from build123d import *

# Parameters (mm, degrees)
F1_DEPTH = 6.35


with BuildPart() as f1:
    # F0 (on Top) → F1 (new body)
    with BuildSketch(Plane.XY):
        with BuildLine():
            ThreePointArc((57.94375, -25.976370723), (48.024670033, -14.636026826), (44.45, 0))
            ThreePointArc((44.45, 0), (0, -44.45), (-44.45, 0))
            ThreePointArc((-44.45, 0), (-48.024670033, -14.636026826), (-57.94375, -25.976370723))
            ThreePointArc((-57.94375, -25.976370723), (-53.0122296555, -34.9564515783), (-46.7007710297, -43.0265962543))
            ThreePointArc((-46.7007710297, -43.0265962543), (-46.1408199964, -43.6066686624), (-45.5932687094, -44.1984597966))
            ThreePointArc((-45.5932687094, -44.1984597966), (0, -63.5), (45.5932687094, -44.1984597966))
            ThreePointArc((45.5932687094, -44.1984597966), (46.1408199964, -43.6066686624), (46.7007710297, -43.0265962543))
            ThreePointArc((46.7007710297, -43.0265962543), (53.0122296555, -34.9564515783), (57.94375, -25.976370723))
        make_face()
        with BuildLine():
            ThreePointArc((57.94375, 25.976370723), (48.024670033, 14.636026826), (44.45, 0))
            Line((44.45, 0), (63.5, 0))
            ThreePointArc((63.5, 0), (62.0954029096, 13.2819779212), (57.94375, 25.976370723))
        make_face()
        with BuildLine():
            ThreePointArc((-44.45, 0), (0, 44.45), (44.45, 0))
            ThreePointArc((44.45, 0), (48.024670033, 14.636026826), (57.94375, 25.976370723))
            ThreePointArc((57.94375, 25.976370723), (53.0122296555, 34.9564515783), (46.7007710297, 43.0265962543))
            ThreePointArc((46.7007710297, 43.0265962543), (46.1408199964, 43.6066686624), (45.5932687094, 44.1984597966))
            ThreePointArc((45.5932687094, 44.1984597966), (0, 63.5), (-45.5932687094, 44.1984597966))
            ThreePointArc((-45.5932687094, 44.1984597966), (-46.1408199964, 43.6066686624), (-46.7007710297, 43.0265962543))
            ThreePointArc((-46.7007710297, 43.0265962543), (-53.0122296555, 34.9564515783), (-57.94375, 25.976370723))
            ThreePointArc((-57.94375, 25.976370723), (-48.024670033, 14.636026826), (-44.45, 0))
        make_face()
        with BuildLine():
            Line((63.5, 0), (44.45, 0))
            ThreePointArc((44.45, 0), (48.024670033, -14.636026826), (57.94375, -25.976370723))
            ThreePointArc((57.94375, -25.976370723), (62.0954029096, -13.2819779212), (63.5, 0))
        make_face()
        with BuildLine():
            ThreePointArc((-57.94375, -25.976370723), (-48.024670033, -14.636026826), (-44.45, 0))
            Line((-44.45, 0), (-63.5, 0))
            ThreePointArc((-63.5, 0), (-62.0954029096, -13.2819779212), (-57.94375, -25.976370723))
        make_face()
        with BuildLine():
            Line((-63.5, 0), (-44.45, 0))
            ThreePointArc((-44.45, 0), (-48.024670033, 14.636026826), (-57.94375, 25.976370723))
            ThreePointArc((-57.94375, 25.976370723), (-62.0954029096, 13.2819779212), (-63.5, 0))
        make_face()
        with BuildLine():
            ThreePointArc((76.2, -12.7), (67.2197438789, -8.9802561211), (63.5, 0))
            ThreePointArc((63.5, 0), (62.0954029096, -13.2819779212), (57.94375, -25.976370723))
            ThreePointArc((57.94375, -25.976370723), (65.6047024614, -29.9299543947), (74.0468101417, -31.6769044168))
            ThreePointArc((74.0468101417, -31.6769044168), (75.1239218386, -31.6982296864), (76.2, -31.75))
            Line((76.2, -31.75), (76.2, -12.7))
        make_face()
        with BuildLine():
            ThreePointArc((57.94375, 25.976370723), (62.0954029096, 13.2819779212), (63.5, 0))
            ThreePointArc((63.5, 0), (67.2197438789, 8.9802561211), (76.2, 12.7))
            Line((76.2, 12.7), (76.2, 31.75))
            ThreePointArc((76.2, 31.75), (75.1239218386, 31.6982296864), (74.0468101417, 31.6769044168))
            ThreePointArc((74.0468101417, 31.6769044168), (65.6047024614, 29.9299543947), (57.94375, 25.976370723))
        make_face()
        with BuildLine():
            ThreePointArc((46.7007710297, 43.0265962543), (53.0122296555, 34.9564515783), (57.94375, 25.976370723))
            ThreePointArc((57.94375, 25.976370723), (65.6047024614, 29.9299543947), (74.0468101417, 31.6769044168))
            ThreePointArc((74.0468101417, 31.6769044168), (59.2262146143, 34.5867715285), (46.7007710297, 43.0265962543))
        make_face()
        with BuildLine():
            ThreePointArc((74.0468101417, -31.6769044168), (65.6047024614, -29.9299543947), (57.94375, -25.976370723))
            ThreePointArc((57.94375, -25.976370723), (53.0122296555, -34.9564515783), (46.7007710297, -43.0265962543))
            ThreePointArc((46.7007710297, -43.0265962543), (59.2262146143, -34.5867715285), (74.0468101417, -31.6769044168))
        make_face()
        with BuildLine():
            ThreePointArc((-76.2, 12.7), (-67.2197438789, 8.9802561211), (-63.5, 0))
            ThreePointArc((-63.5, 0), (-62.0954029096, 13.2819779212), (-57.94375, 25.976370723))
            ThreePointArc((-57.94375, 25.976370723), (-65.6047024614, 29.9299543947), (-74.0468101417, 31.6769044168))
            ThreePointArc((-74.0468101417, 31.6769044168), (-75.1239218386, 31.6982296864), (-76.2, 31.75))
            Line((-76.2, 31.75), (-76.2, 12.7))
        make_face()
        with BuildLine():
            ThreePointArc((-57.94375, -25.976370723), (-62.0954029096, -13.2819779212), (-63.5, 0))
            ThreePointArc((-63.5, 0), (-67.2197438789, -8.9802561211), (-76.2, -12.7))
            Line((-76.2, -12.7), (-76.2, -31.75))
            ThreePointArc((-76.2, -31.75), (-75.1239218386, -31.6982296864), (-74.0468101417, -31.6769044168))
            ThreePointArc((-74.0468101417, -31.6769044168), (-65.6047024614, -29.9299543947), (-57.94375, -25.976370723))
        make_face()
        with BuildLine():
            ThreePointArc((-74.0468101417, 31.6769044168), (-65.6047024614, 29.9299543947), (-57.94375, 25.976370723))
            ThreePointArc((-57.94375, 25.976370723), (-53.0122296555, 34.9564515783), (-46.7007710297, 43.0265962543))
            ThreePointArc((-46.7007710297, 43.0265962543), (-59.2262146143, 34.5867715285), (-74.0468101417, 31.6769044168))
        make_face()
        with BuildLine():
            ThreePointArc((-46.7007710297, -43.0265962543), (-53.0122296555, -34.9564515783), (-57.94375, -25.976370723))
            ThreePointArc((-57.94375, -25.976370723), (-65.6047024614, -29.9299543947), (-74.0468101417, -31.6769044168))
            ThreePointArc((-74.0468101417, -31.6769044168), (-59.2262146143, -34.5867715285), (-46.7007710297, -43.0265962543))
        make_face()
        with BuildLine():
            Line((76.2, 31.75), (76.2, 12.7))
            ThreePointArc((76.2, 12.7), (85.1802561211, 8.9802561211), (88.9, 0))
            ThreePointArc((88.9, 0), (85.1802561211, -8.9802561211), (76.2, -12.7))
            Line((76.2, -12.7), (76.2, -31.75))
            ThreePointArc((76.2, -31.75), (98.6506403027, -22.4506403027), (107.95, 0))
            ThreePointArc((107.95, 0), (98.6506403027, 22.4506403027), (76.2, 31.75))
        make_face()
        with BuildLine():
            ThreePointArc((-76.2, -12.7), (-88.9, 0), (-76.2, 12.7))
            Line((-76.2, 12.7), (-76.2, 31.75))
            ThreePointArc((-76.2, 31.75), (-107.95, 0), (-76.2, -31.75))
            Line((-76.2, -31.75), (-76.2, -12.7))
        make_face()
    extrude(amount=F1_DEPTH)


solid = f1.part
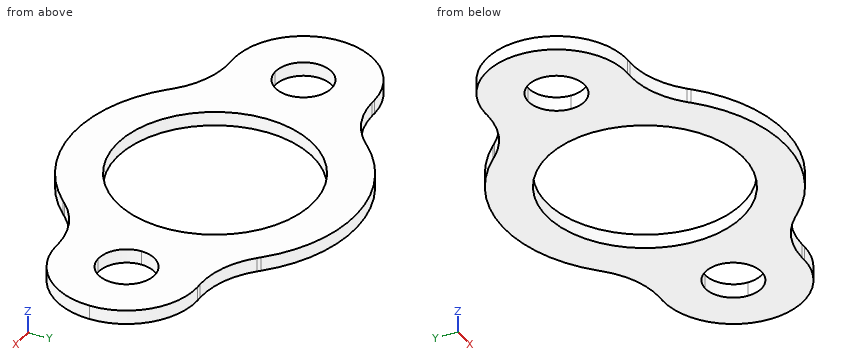
Check sheet for the modelled part. Datum: model origin and axes. Units: mm. Coordinates: 2 decimals unless noted, no trailing zeros. Loops run counter-clockwise (first coordinate to the right, second up) from the corner with the lowest first, then second, coordinate; pieces in that order, holes last. Notation, with made-up numbers: (14.25, 13.25) -> (50.25, 13.25) arc R26 cw to (50.25, 41.25) -> close; hole circle Ø7 at (-27.5, 50.5). An arc over 180 degrees is marked (long way). Write item = value, one per line. Start each with the question number.
1. Depth check by flat-ended pin: P1, Ø1.5, axis at x = 62.5, z = 1, coming from the -Y side; P2, Ø1.5, axis at y = -23.5, z = 5, coming from the +X side; P3, Ø6, axis at x = 31.5, y = 25, coming from the +Z side. Enter the tip coordinate at first touch or a pass-through.
2. Section check A-A on x = 0. Record the cut outline in (y, z), then the cut area to 3 significant figures.
3. Section check B-B on z = 4.5. Record the cut outline in (x, y).
4. Material ranges on line 1 (X direction, y = 9, z = 4.25); line 2 (X direction, y = 9.5, z = 1.5); line 3 (X direction, y = -41, z = 6.25), recorded low to high.
5. Section check D-D on x = 93.5. Record the cut outline in (y, z).
6. Section check C-C on y = 34.5. Record the cut outline in (x, z), then the cut area to 3 significant figures.
Responses:
q1.P1 = -33.64
q1.P2 = 98.35
q1.P3 = through
q2.outline = (-63.5, 0) -> (-44.45, 0) -> (-44.45, 6.35) -> (-63.5, 6.35) -> close; (44.45, 0) -> (63.5, 0) -> (63.5, 6.35) -> (44.45, 6.35) -> close
q2.area = 242 mm2
q3.outline = (-76.2, -31.75) arc R38.1 cw to (-45.59, -44.2) arc R63.5 ccw to (45.59, -44.2) arc R38.1 cw to (76.2, -31.75) arc R31.75 ccw to (76.2, 31.75) arc R38.1 cw to (45.59, 44.2) arc R63.5 ccw to (-45.59, 44.2) arc R38.1 cw to (-76.2, 31.75) arc R31.75 ccw to start; hole circle Ø25.4 at (-76.2, 0); hole circle Ø88.9 at (0, 0); hole circle Ø25.4 at (76.2, 0)
q4.line_1 = -106.65 to -85.16, -67.24 to -43.53, 43.53 to 67.24, 85.16 to 106.65
q4.line_2 = -106.5 to -84.63, -67.77 to -43.42, 43.42 to 67.77, 84.63 to 106.5
q4.line_3 = -48.86 to -17.17, 17.17 to 48.86
q5.outline = (-26.62, 0) -> (26.62, 0) -> (26.62, 6.35) -> (-26.62, 6.35) -> close
q6.outline = (-59.44, 0) -> (-28.03, 0) -> (-28.03, 6.35) -> (-59.44, 6.35) -> close; (28.03, 0) -> (59.44, 0) -> (59.44, 6.35) -> (28.03, 6.35) -> close
q6.area = 399 mm2
